```python
from build123d import *

# Parameters (mm, degrees)
BOSS_EXTRUDE1_DEPTH     = 16
SKETCH2_W               = 22
SKETCH2_H               = 15
CUT_EXTRUDE1_DEPTH      = 12
CUT_EXTRUDE2_DEPTH      = 94.037626797
CUT_EXTRUDE2_DEPTH_BACK = 12
CUT_EXTRUDE4_DEPTH      = 12


with BuildPart() as part:
    # Sketch1 → Boss-Extrude1 (new body)
    with BuildSketch(Plane(origin=(0, 0, 0), x_dir=(1, 0, 0), z_dir=(0, 1, 0))):
        Polygon((69.282032303, 0), (34.641016151, 60), (-34.641016151, 60), (-69.282032303, 0), (-34.641016151, -60), (34.641016151, -60), align=None)
    extrude(amount=BOSS_EXTRUDE1_DEPTH)

    # Sketch2 → Cut-Extrude1 (cut)
    with BuildSketch(Plane(origin=(0, 16, 0), x_dir=(1, 0, 0), z_dir=(0, 1, 0))):
        with Locations((-18.641016151, 52.5)):
            Rectangle(SKETCH2_W, SKETCH2_H)
        with Locations((18.641016151, 52.5)):
            Rectangle(SKETCH2_W, SKETCH2_H)
        Polygon((66.782032303, -4.330127019), (53.791651246, 3.169872981), (42.791651246, -15.882685902), (55.782032303, -23.382685902), align=None)
        Polygon((48.141016151, -36.617314098), (35.150635095, -29.117314098), (24.150635095, -48.169872981), (37.141016151, -55.669872981), align=None)
        Polygon((-37.141016151, -55.669872981), (-24.150635095, -48.169872981), (-35.150635095, -29.117314098), (-48.141016151, -36.617314098), align=None)
        Polygon((-55.782032303, -23.382685902), (-42.791651246, -15.882685902), (-53.791651246, 3.169872981), (-66.782032303, -4.330127019), align=None)
    extrude(amount=-CUT_EXTRUDE1_DEPTH, mode=Mode.SUBTRACT)

    # Sketch3 → Cut-Extrude2 (cut, two sides: drawn at the far end of the back side and taken through both)
    with BuildSketch(Plane(origin=(0, 16, 0), x_dir=(1, 0, 0), z_dir=(0, 1, 0)).offset(-CUT_EXTRUDE2_DEPTH_BACK)):
        Polygon((-43.560889132, -5.4496732), (17.060889132, -40.4496732), (43.560889132, 5.4496732), (-17.060889132, 40.4496732), align=None)
        Polygon((-22.060889132, 31.789419162), (-28.060889132, 21.397114317), (-49.711524227, 33.897114317), (-43.711524227, 44.289419162), align=None)
    extrude(amount=CUT_EXTRUDE2_DEPTH + CUT_EXTRUDE2_DEPTH_BACK, mode=Mode.SUBTRACT)

    # Sketch4 → Cut-Extrude4 (cut)
    with BuildSketch(Plane(origin=(0, 16, 0), x_dir=(1, 0, 0), z_dir=(0, 1, 0))):
        Polygon((-53.791651246, 3.169872981), (-59.853829072, -0.330127019), (-64.663230149, 8), (-60.621778265, 15), align=None)
        Polygon((-24.150635095, -48.169872981), (-30.212812921, -51.669872981), (-25.403411844, -60), (-17.320508076, -60), align=None)
        Polygon((43.301270189, 45), (29.641016151, 45), (29.641016151, 52), (39.259818305, 52), align=None)
        Polygon((-43.301270189, 45), (-29.641016151, 45), (-29.641016151, 52), (-39.259818305, 52), align=None)
        Polygon((17.320508076, -60), (24.150635095, -48.169872981), (30.212812921, -51.669872981), (25.403411844, -60), align=None)
        Polygon((60.621778265, 15), (53.791651246, 3.169872981), (59.853829072, -0.330127019), (64.663230149, 8), align=None)
    extrude(amount=-CUT_EXTRUDE4_DEPTH, mode=Mode.SUBTRACT)


solid = part.part
```
Geometry check sheet. Reference: the model listing, model coordinates, mm. A direction names the side the tool comes from. Round coordinates to 2 decimals unless told otherwise and drop trailing zeros. Order: outer loops, then holes, each group sorted by start corner. A loop starts at its lowest first (then second) coordinate and runs counter-clockwise, first axis right, second up. Notation, with made-up numbers: (-13, 84.25) -> (0, 84.25) arc R15 ccw to (0, 100.25) -> close; hole circle Ø8 at (47, 10). An arc over 180 degrees is marked (long way). Return JSON: item names as keys, results as strings. Group by question number.
Q1. Tool access check on faces 1 (the flat face through (-26, 10, -45)), 2 (the flat face through (29.641, 10, -56)), 3 (the flat face through (-62.225, 10.084, -3.777)). Record the directions out of +Z, -Z, +X, -X, +Y, -Y that give a thin tool (end or side, any length) a straight path to the whole face; none if there is none.
Q2. Section check B-B, the plane z = 46. Record the boundary of the cut face in (x, y), plus the area to 3 significant figures.
Q3. Gauge pin test, flat ends, axial feed: pin 1 (3.5 mm diameter, centred on y = 12, z = -51.5, fed in from +X); pin 2 (9 mm diameter, centred on y = 9, z = -58, fed in from +X); pin 3 (3 mm diameter, centred on x = -21.5, y = 12.5, fed in from -Z). Record the tip position at first contact, or that the pin passes through.
Q4. Section check A-A, the plane y = 2. Record the boundary of the cut face in (x, z), plus the area to 3 significant figures.
Q5. Section check C-C, the plane y = 13. Count the separate pieces of the cut face and the enclosed holes in it, plus the area to 3 significant figures.
Q6. Release check for a two-part mould opening along Z. For faces 4 (the flat face through (-51.72, 6.11, -30.42)), 5 (the flat face through (-27.84, 10.08, 55.78)), 6 (the flat face through (-65, 16, -1)), 7 (the flat face through (-52.204, 6.11, 29.58)) record: released by +Z, released by -Z, zero draft, split by the parting line, or undercut.
Q7. Section check D-D, the plane x = -15. Record the boundary of the cut face in (y, z), plus the area to 3 significant figures.
Q8. Material ranges on probe 1 along X at (y, z) = (4.25, 53.5); probe 2 along Y at (x, z) = (15, -9); probe 3 along Z at (x, y) = (17, 4.25), recorded low to high. Write a range as from..to.
Numbers:
{
 "1": {"face 1": "-X, +Y", "face 2": "-Z, +Y", "face 3": "+Y"},
 "2": {"outline": "(-42.72, 0) -> (42.72, 0) -> (42.72, 4) -> (25.4, 4) -> (25.4, 16) -> (-25.4, 16) -> (-25.4, 4) -> (-42.72, 4) -> close", "area": "951 mm^2"},
 "3": {"pin 1": "x = 39.26", "pin 2": "x = 38.39", "pin 3": "z = -45"},
 "4": {"outline": "(-69.28, 0) -> (-34.64, -60) -> (34.64, -60) -> (69.28, 0) -> (34.64, 60) -> (-34.64, 60) -> close", "area": "12,500 mm^2"},
 "5": {"separate pieces": "7", "enclosed holes": "0", "area": "5,990 mm^2"},
 "6": {"face 4": "released by -Z", "face 5": "undercut", "face 6": "zero draft", "face 7": "released by +Z"},
 "7": {"outline": "(0, -60) -> (4, -60) -> (4, -45) -> (16, -45) -> (16, -39.26) -> (4, -39.26) -> (4, 21.94) -> (16, 21.94) -> (16, 60) -> (0, 60) -> close", "area": "1,010 mm^2"},
 "8": {"probe 1": "-33.38..-29.16, -21.07..21.07, 29.16..33.38", "probe 2": "0..4", "probe 3": "-45..-20.78, 40.41..60"}
}
